Source: CAD feature listing. Evaluate the final solid. Frame: model axes, mm. A direction names the side the tool comes from. Round coordinates to 2 decimals unless told otherwise and drop trailing zeros. Write each loop counter-clockwise with the first axis right and the second up, starting at its lowest first coordinate (ties: lowest second). Pieces come first, ordered by that corner, then holes. Notation, with made-up numbers: M -40,56 L -29,56 A16 ccw -29,81 Z; hole C 79.25,89.5 d5. An arc over 180 degrees is marked long. Use a Markdown table: item, result.
Autodesk Inventor part; units mm, degrees
ref_plane "YZ Plane" through (0, 0, 0) normal (1, 0, 0) x (0, 1, 0)
ref_plane "XZ Plane" through (0, 0, 0) normal (0, 1, 0) x (-1, 0, 0)
ref_plane "XY Plane" through (0, 0, 0) normal (0, 0, 1) x (1, 0, 0)
sketch "Sketch1" plane through (0, 0, 0) normal (0, 1, 0) x (-1, 0, 0)
  circle A0 centre (0, 0) radius 70
  dimension "d0" = 140
extrude "Extrusion1" add sketch "Sketch1" along normal blind 28
sketch "Sketch2" plane through (0, 28, 0) normal (0, 1, 0) x (1, 0, 0)
  circle A0 centre (0, 0) radius 8.25
  dimension "d3" = 16.5
extrude "Extrusion2" cut sketch "Sketch2" against normal blind 28
sketch "Sketch3" plane through (0, 28, 0) normal (0, 1, 0) x (1, 0, 0)
  circle A0 centre (0, 0) radius 8.25
  circle A1 centre (0, 0) radius 65
  circle A2 centre (0, 0) radius 10.5
  dimension "d6" = 130
  dimension "d7" = 21
extrude "Extrusion3" cut sketch "Sketch3" against normal blind 25 contours A1
sketch "Sketch4" plane through (0, 3, 0) normal (0, 1, 0) x (1, 0, 0)
  line L0 (-77.4845, 0) -> (88.5537, 0)
  line L1 (88.5537, 0) -> (88.5537, 100.8261)
  line L2 (88.5537, 100.8261) -> (-77.4845, 100.8261)
  line L3 (-77.4845, 100.8261) -> (-77.4845, 0)
  point P0 (0, 0)
  point P1 (0, 0)
extrude "Extrusion4" cut sketch "Sketch4" along normal blind 220
sketch "Sketch5" plane through (0, 3, 0) normal (0, 1, 0) x (1, 0, 0)
  arc A0 (-10.5, 0) -> (10.5, 0) centre (0, 0) ccw
  arc A1 (-65, 0) -> (65, 0) centre (0, 0) ccw
  arc A2 (-10.5, 0) -> (10.5, 0) centre (0, 0) ccw
  line L0 (10.5, 0) -> (10.5, -64.1463)
  line L1 (-10.5, 0) -> (-10.5, -64.1463)
  arc A3 (-10.5, -64.1463) -> (10.5, -64.1463) centre (0, 0) ccw
  arc A4 (-10.5, 0) -> (10.5, 0) centre (0, 0) ccw
extrude "Extrusion5" add sketch "Sketch5" along normal blind 3
sketch "Sketch6" plane through (0, 28, 0) normal (0, 1, 0) x (1, 0, 0)
  line L0 (-8.25, 0) -> (-10.5, 0)
  line L1 (-8.25, 0) -> (8.25, 0)
  line L2 (8.25, 0) -> (8.25, 75.2128)
  line L3 (8.25, 75.2128) -> (-8.25, 75.2128)
  line L4 (-8.25, 75.2128) -> (-8.25, 0)
  point P0 (0, 0)
  dimension "d14" = 16.5
extrude "Extrusion6" cut sketch "Sketch6" against normal blind 30
sketch "Sketch8" plane through (0, 3, 0) normal (0, 1, 0) x (1, 0, 0)
  arc A0 (-65, 0) -> (65, 0) centre (0, 0) ccw
  line L0 (65, 0) -> (70, 0)
  arc A1 (70, 0) -> (-70, 0) centre (0, 0) ccw
  line L1 (-70, 0) -> (-65, 0)
  arc A2 (-10.5, 0) -> (10.5, 0) centre (0, 0) ccw
  line L2 (-10.5, 0) -> (-8.25, 0)
  arc A3 (8.25, 0) -> (-8.25, 0) centre (0, 0) ccw
  line L3 (8.25, 0) -> (10.5, 0)
  circle A4 centre (0, 0) radius 8.25
  arc A5 (65, 0) -> (-65, 0) centre (0, 0) ccw
  line L4 (-65, 0) -> (-70, 0)
  line L5 (65, 0) -> (70, 0)
  arc A6 (70, 0) -> (-70, 0) centre (0, 0) ccw
  arc A7 (70, 0) -> (70, 0) centre (0, 0) ccw
extrude "Extrusion7" cut sketch "Sketch8" against normal blind 30 contours L1 A1 L0 A5
fillet "Fillet1" radius 3 1 edges at (0, 6, 10.5)
fillet "Fillet2" radius 3 1 edges at (0, 0, 70)
fillet "Fillet4" radius 3 1 edges at (0, 28, 70)
sketch "Sketch11" plane through (0, 28, 0) normal (0, 1, 0) x (1, 0, 0)
  line L0 (-65, 0) -> (-67.69, 0)
  line L1 (-64.8074, 5) -> (-67.4974, 5)
  arc A0 (-67.5051, 5) -> (-67.69, 0) centre (0, 0) ccw
  arc A1 (-64.8074, 5) -> (-65, 0) centre (0, 0) ccw
  line L2 (-65, 0) -> (-67.69, 0)
  line L3 (-70, 0) -> (-67, 0)
  line L4 (-64.8074, 5) -> (-67.5051, 5)
  dimension "d30" = 2.69
  dimension "d32" = 2.69
extrude "Extrusion10" add sketch "Sketch11" against normal blind 28
mirror "Mirror3" about plane through (0, 0, 0) normal (1, 0, 0) of "Extrusion10"
properties part number "casept2"
Q1. Reachability of faces 4 (the flat face through (-1, 0, 15)), 5 (the cylindrical face through (67.645, 14.196, -2.467)), 6 (the flat face through (8.25, 2, -32)), 7 (the flat face through (10.5, 5, 32)), 8 (the cylindrical face through (64.953, 15.675, -2.467)) from +Z, -Z, +X, -X, +Y, -Y: full face, straight path, thin tool, end or side. Return the list, or none.
Results are:
| item | result |
|---|---|
| face 4 | +Z, -Z, +X, -X, -Y |
| face 5 | -Z, +X, +Y, -Y |
| face 6 | -Z, +Y, -Y |
| face 7 | -Z, +Y |
| face 8 | +Y |
Q2. Mould query, pull axis X, two halves, no side actions, for faces 1 (the cylindrical face through (-0.2, 18.6, 10.5)), 2 (the cylindrical face through (47.53, 1.52, -44.34)), 3 (the flat face through (0.8, 28, 8.4)). Classes: +X half, -X half, draft (parallel to the pull), parting line (faces both ways), or undercut.
Results are:
| item | result |
|---|---|
| face 1 | undercut |
| face 2 | +X half |
| face 3 | draft |
Q3. Line query: L1, parallel to X at y = 23, z = 9.5; L2, parallel to X at y = 3.5, z = 60.5; L3, parallel to Y at x = 60, z = -13. Output: solid intervals per line, ascending.
Results are:
| item | result |
|---|---|
| L1 | -69.35 to -64.3, -4.47 to 4.47, 64.3 to 69.35 |
| L2 | -35.21 to -23.76, -10.5 to 10.5, 23.76 to 35.21 |
| L3 | 0 to 3 |
Q4. First-contact query: pin 1 Ø1.5 at (x, z) = (41, -46) entering from -Y; pin 2 Ø0.8 at (x, y) = (65.5, 20) entering from -Z; pin 3 Ø3 at (x, y) = (-53, 13.5) entering from +Z; pin 4 Ø0.7 at (x, y) = (-9.5, 10) entering from -Z. Flat tips, straight axial feed; report the tip coordinate or a pass-through.
Results are:
| item | result |
|---|---|
| pin 1 | y = 0 |
| pin 2 | z = -5 |
| pin 3 | z = 47.41 |
| pin 4 | z = 0 |
Q5. Section A-A on x = 0. Return loops of the section in (y, z).
Results are:
| item | result |
|---|---|
| outline | M 0,8.25 L 28,8.25 L 28,10.5 L 9,10.5 A3 cw 6,13.5 L 6,65 L 28,65 L 28,67 A3 ccw 25,70 L 3,70 A3 ccw 0,67 Z |
